from build123d import *

# Parameters (mm, degrees)
SKETCH1_W           = 10
SKETCH1_H           = 10
BOSS_EXTRUDE1_DEPTH = 24
SKETCH2_W           = 3
SKETCH2_H           = 3
BOSS_EXTRUDE2_DEPTH = 10
SKETCH3_R           = 0.5
BOSS_EXTRUDE3_DEPTH = 10


with BuildPart() as part:
    # Sketch1 → Boss-Extrude1 (new body)
    with BuildSketch(Plane.XY):
        Rectangle(SKETCH1_W, SKETCH1_H)
    extrude(amount=BOSS_EXTRUDE1_DEPTH)

    # Sketch2 → Boss-Extrude2 (add)
    with BuildSketch(Plane.XY.offset(24)):
        Rectangle(SKETCH2_W, SKETCH2_H)
    extrude(amount=BOSS_EXTRUDE2_DEPTH)

    # Sketch3 → Boss-Extrude3 (add)
    with BuildSketch(Plane.XZ.offset(5)):
        with Locations(Location((-3.81, 10.415606067, 0), (0, 0, 90))):
            Circle(SKETCH3_R)
        with Locations(Location((3.81, 10.415606067, 0), (0, 0, 90))):
            Circle(SKETCH3_R)
        with Locations(Location((3.81, 7.875606067, 0), (0, 0, 90))):
            Circle(SKETCH3_R)
        with Locations(Location((3.81, 5.335606067, 0), (0, 0, 90))):
            Circle(SKETCH3_R)
        with Locations(Location((-3.81, 7.875606067, 0), (0, 0, 90))):
            Circle(SKETCH3_R)
        with Locations(Location((-3.81, 5.335606067, 0), (0, 0, 90))):
            Circle(SKETCH3_R)
    extrude(amount=BOSS_EXTRUDE3_DEPTH)


solid = part.part
Model file for the job. Use its own axes, mm. A direction names the side the tool comes from. Give positions to 0.01 mm unless a question says otherwise; leave off trailing zeros. Write each loop counter-clockwise with the first axis right and the second up, starting at its lowest first coordinate (ties: lowest second). Pieces come first, ordered by that corner, then holes. Notation, with made-up numbers: (2, 83.25) -> (54, 83.25) arc R30 cw to (54, 114.25) -> close; hole circle Ø2 at (4, 10.25). An arc over 180 degrees is marked (long way). Write item = value, one per line.
(1) Slice it at D-D, the plane z = 16. Give the cut face in (x, y).
Determined:
outline = (-5, -5) -> (5, -5) -> (5, 5) -> (-5, 5) -> close
(2) Slice it at A-A, the plane y = -11. Give the cut face in (x, z).
Determined:
outline = circle Ø1 at (-3.81, 5.34); circle Ø1 at (-3.81, 7.88); circle Ø1 at (-3.81, 10.42); circle Ø1 at (3.81, 5.34); circle Ø1 at (3.81, 7.88); circle Ø1 at (3.81, 10.42)
(3) Slice it at B-B, the plane y = 0. Give the cut face in (x, z), then the cut area to 3 significant figures.
Determined:
outline = (-5, 0) -> (5, 0) -> (5, 24) -> (1.5, 24) -> (1.5, 34) -> (-1.5, 34) -> (-1.5, 24) -> (-5, 24) -> close
area = 270 mm2
(4) Probe line 1 along Z through (x, y) = (4.25, -8); line 2 along Y through (x, z) = (-3.5, 2); line 3 along Z through (x, y) = (-2.5, -1). List the from-to ranges inside material, lowest first.
Determined:
line_1 = 5.1 to 5.57, 7.64 to 8.11, 10.18 to 10.65
line_2 = -5 to 5
line_3 = 0 to 24
(5) Tool access for faces 4 (the face through (-4, -15, 8)), 5 (the face through (-4.306, -9.93, 7.811)), 6 (the face through (0, 1.5, 29)), 7 (the face through (0, -1.5, 29)): list every direction of +Z, -Z, +X, -X, +Y, -Y with a clear straight run to the whole face (end or side of a thin tool).
Determined:
face_4 = +Z, -Z, +X, -X, -Y
face_5 = -Y
face_6 = +Z, +X, -X, +Y
face_7 = +Z, +X, -X, -Y
(6) Flat gauge pins, fed straight in: P1, Ø1.5, axis at x = 0.5, z = 30.5, coming from the +Y side; P2, Ø3, axis at x = 0, y = 2, coming from the +Z side; P3, Ø3.5, axis at x = 0.5, z = 27, coming from the -Y side; P4, Ø1.5, axis at y = 0, z = 28, coming from the +X side. Where does each tip first touch, or does it go through?
Determined:
P1 = 1.5
P2 = 34
P3 = -1.5
P4 = 1.5
(7) Mould opens along X. For faces 1 (the face through (-5, 0, 12)), 2 (the face through (0, 5, 12)), 3 (the face through (3.314, -9.93, 10.351)) say: released by +X, released by -X, zero draft, split by the parting line, or undercut.
Determined:
face_1 = released by -X
face_2 = zero draft
face_3 = undercut
